Design review of the part built by this model. Coordinates are the model's own, in mm. A direction names the side the tool comes from. Coordinates: 2 decimals unless noted, no trailing zeros. Loops run counter-clockwise (first coordinate to the right, second up) from the corner with the lowest first, then second, coordinate; pieces in that order, holes last. Notation, with made-up numbers: M 68,-13.75 L 100,-13.75 A30 ccw 100,25.25 Z; hole C -27,35.25 d6. An arc over 180 degrees is marked long. Answer as a JSON object with one key per item and string values. Group by question number.
1. Draft analysis for pull direction Z (two halves, no side actions). For faces 1 (the flat face through (-21, 16, 0)), 2 (the conical face through (-2, 57, 0)), 3 (the flat face through (16, 28, -16)), state which applies: +Z half, -Z half, draft (parallel to the pull), parting line (faces both ways), or undercut.
2. Consider section D-D (z = 0). State the section outline as (x, y) points.
3. Machinability: for faces 4 (the flat face through (0, 16, -21)), 5 (the cylindrical face through (15.57, 30.54, 14)), which of the approach directions +Z, -Z, +X, -X, +Y, -Y give a long, thin tool a straight path to every point of the face, cutting with its end or side? Answer none if there is none.
4. Consider section C-C (x = 0). State the section outline as (y, z) points.
5. Consider section A-A (x = 15.5). State the section outline as (y, z) points.
6. Insertion check: pin 1 (1 mm diameter, centred on x = -7, z = 1.5, fed in from +Y); pin 2 (1.8 mm diameter, centred on x = -15.5, z = 15.5, fed in from +Y); pin 3 (3.5 mm diameter, centred on x = -15.5, z = -15.5, fed in from +Y). Each pin has a flat end and moves straight along its axis. Give the tip position at first contact, or say it passes through.
7. Consider section B-B (z = -15.5). State the section outline as (x, y) points, then the cut area to 3 significant figures.
8. To check wall thickness, follow probe 1 along X at (y, z) = (29.6, -15.5); probe 2 along X at (y, z) = (29, -15). State the ranges of each line that lie inside material, in increasing order.
from build123d import *

# Parameters (mm, degrees)
SKETCH1_W           = 42
SKETCH1_H           = 42
BOSS_EXTRUDE1_DEPTH = 33
SKETCH2_R           = 11
BOSS_EXTRUDE2_DEPTH = 2
SKETCH3_R           = 2.5
BOSS_EXTRUDE3_DEPTH = 22.25
CHAMFER1_SIZE       = 3.6
SKETCH4_R           = 1.5
CUT_EXTRUDE1_DEPTH  = 5
CHAMFER2_SIZE       = 0.75


with BuildPart() as part:
    # Sketch1 → Boss-Extrude1 (new body)
    with BuildSketch(Plane(origin=(0, 0, 0), x_dir=(1, 0, 0), z_dir=(0, 1, 0))):
        Rectangle(SKETCH1_W, SKETCH1_H)
    extrude(amount=BOSS_EXTRUDE1_DEPTH)

    # Sketch2 → Boss-Extrude2 (add)
    with BuildSketch(Plane(origin=(0, 33, 0), x_dir=(1, 0, 0), z_dir=(0, 1, 0))):
        with Locations(Location((0, 0, 0), (0, 0, 270))):
            Circle(SKETCH2_R)
    extrude(amount=BOSS_EXTRUDE2_DEPTH)

    # Sketch3 → Boss-Extrude3 (add)
    with BuildSketch(Plane(origin=(0, 35, 0), x_dir=(1, 0, 0), z_dir=(0, 1, 0))):
        with Locations(Location((0, 0, 0), (0, 0, 270))):
            Circle(SKETCH3_R)
    extrude(amount=BOSS_EXTRUDE3_DEPTH)

    # Chamfer1
    chamfer1_edges = [part.edges().sort_by_distance(p)[0] for p in [
        (21, 16.5, 21),
        (-21, 16.5, 21),
        (-21, 16.5, -21),
        (21, 16.5, -21),
    ]]
    chamfer(chamfer1_edges, length=CHAMFER1_SIZE)

    # Sketch4 → Cut-Extrude1 (cut)
    with BuildSketch(Plane(origin=(0, 33, 0), x_dir=(1, 0, 0), z_dir=(0, 1, 0))):
        with Locations(Location((15.5, 15.5, 0), (0, 0, 270))):
            Circle(SKETCH4_R)
        with Locations(Location((15.5, -15.5, 0), (0, 0, 270))):
            Circle(SKETCH4_R)
        with Locations(Location((-15.5, -15.5, 0), (0, 0, 270))):
            Circle(SKETCH4_R)
        with Locations(Location((-15.5, 15.5, 0), (0, 0, 270))):
            Circle(SKETCH4_R)
    extrude(amount=-CUT_EXTRUDE1_DEPTH, mode=Mode.SUBTRACT)

    # Chamfer2
    chamfer2_edges = [part.edges().sort_by_distance(p)[0] for p in [
        (0, 57.25, -2.5),
    ]]
    chamfer(chamfer2_edges, length=CHAMFER2_SIZE)


solid = part.part
Findings below:
{
 "1": {"face 1": "draft", "face 2": "parting line", "face 3": "undercut"},
 "2": {"outline": "M -21,0 L 21,0 L 21,33 L 11,33 L 11,35 L 2.5,35 L 2.5,56.5 L 1.75,57.25 L -1.75,57.25 L -2.5,56.5 L -2.5,35 L -11,35 L -11,33 L -21,33 Z"},
 "3": {"face 4": "-Z, +X, -X, +Y, -Y", "face 5": "+Y"},
 "4": {"outline": "M 0,-21 L 33,-21 L 33,-11 L 35,-11 L 35,-2.5 L 56.5,-2.5 L 57.25,-1.75 L 57.25,1.75 L 56.5,2.5 L 35,2.5 L 35,11 L 33,11 L 33,21 L 0,21 Z"},
 "5": {"outline": "M 0,-21 L 33,-21 L 33,-17 L 28,-17 L 28,-14 L 33,-14 L 33,14 L 28,14 L 28,17 L 33,17 L 33,21 L 0,21 Z"},
 "6": {"pin 1": "stops at y = 35", "pin 2": "stops at y = 28", "pin 3": "stops at y = 33"},
 "7": {"outline": "M -21,0 L 21,0 L 21,33 L 17,33 L 17,28 L 14,28 L 14,33 L -14,33 L -14,28 L -17,28 L -17,33 L -21,33 Z", "area": "1,360 mm^2"},
 "8": {"probe 1": "x = -21 to -17, -14 to 14, 17 to 21", "probe 2": "x = -21 to -16.91, -14.09 to 14.09, 16.91 to 21"}
}
